Design review of the part built by this model. Coordinates are the model's own, in mm. A direction names the side the tool comes from. Coordinates: 2 decimals unless noted, no trailing zeros. Loops run counter-clockwise (first coordinate to the right, second up) from the corner with the lowest first, then second, coordinate; pieces in that order, holes last.
Q1. Add section B-B on z = -31. Give the boundary of the cut face in (x, y) (3 decimals), and give its area (3 significant figures).
Q2. Add section A-A on x = 167. Give the boundary of the cut face in (y, z) (3 decimals).
Q3. Draft analysis for pull direction Y (two halves, no side actions). For faces 1 (the face through (691, 22, -44.45)), 2 (the face through (695, 22, -41.275)), 3 (the face through (745, 0, -22)), 4 (the face through (745, 22, -3.175)), state which applies: released by +Y, released by -Y, zero draft, split by the parting line, or undercut.
Q4. Machinability: for faces 5 (the face through (745, 41.275, -22)), 6 (the face through (1444.68, 2.57, -28.87)), which of the approach directions +Z, -Z, +X, -X, +Y, -Y give a long, thin tool a straight path to every point of the face, cutting with its end or side? Answer none if there is none.
Q5. Wall thickness on probe 1 along Z at (x, y) = (1351, 20.5) (3 decimals); probe 2 along Y at (x, z) = (39.37, -2.3): over which ranges is each line inside the solid? List them lowest first.
```python
from build123d import *

# Parameters (mm, degrees)
SKETCH1_W               = 44.45
SKETCH1_H               = 44.45
SKETCH1_W_2             = 38.1
SKETCH1_H_2             = 38.1
BOSS_EXTRUDE1_DEPTH     = 1524
CUT_EXTRUDE1_DEPTH      = 45.45
F_1_4_CLEARANCE_HOLE1_D = 6.7564
CUT_EXTRUDE2_DEPTH      = 45.45


with BuildPart() as part:
    # Sketch1 → Boss-Extrude1 (new body)
    with BuildSketch(Plane(origin=(0, 0, 0), x_dir=(0, 0, -1), z_dir=(1, 0, 0))):
        with Locations((22.225, 22.225)):
            Rectangle(SKETCH1_W, SKETCH1_H)
        with Locations((22.225, 22.225)):
            Rectangle(SKETCH1_W_2, SKETCH1_H_2, mode=Mode.SUBTRACT)
    extrude(amount=BOSS_EXTRUDE1_DEPTH)

    # Sketch2 → Cut-Extrude1 (cut, through all)
    with BuildSketch(Plane(origin=(0, 44.45, 0), x_dir=(1, 0, 0), z_dir=(0, 1, 0))):
        Polygon((1524, 0), (1401.874628705, 44.45), (1524, 44.45), align=None)
    extrude(amount=-CUT_EXTRUDE1_DEPTH, mode=Mode.SUBTRACT)

    # 1/4 Clearance Hole1 (through all)
    with Locations(Plane.XY):
        with Locations((39.37, 22.225)):
            Hole(F_1_4_CLEARANCE_HOLE1_D / 2)

    # Sketch5 → Cut-Extrude2 (cut, through all)
    with BuildSketch(Plane(origin=(0, 44.45, 0), x_dir=(1, 0, 0), z_dir=(0, 1, 0))):
        Polygon((1524, 0), (1511.3, 0), (1511.3, 4.622421975), align=None)
    extrude(amount=-CUT_EXTRUDE2_DEPTH, mode=Mode.SUBTRACT)


solid = part.part
```
Entries:
1. outline: (0, 0) - (1438.828, 0) - (1438.828, 3.175) - (0, 3.175) - close; (0, 41.275) - (1438.828, 41.275) - (1438.828, 44.45) - (0, 44.45) - close
1. area: 9,140 mm2
2. outline: (0, -44.45) - (44.45, -44.45) - (44.45, 0) - (0, 0) - close; hole (3.175, -41.275) - (41.275, -41.275) - (41.275, -3.175) - (3.175, -3.175) - close
3. face 1: zero draft
3. face 2: undercut
3. face 3: released by -Y
3. face 4: undercut
4. face 5: +X, -X
4. face 6: -Z, +X, +Y, -Y
5. probe 1: z = -44.45 to -41.275, -3.175 to 0
5. probe 2: y = 0 to 18.85, 25.6 to 44.45
